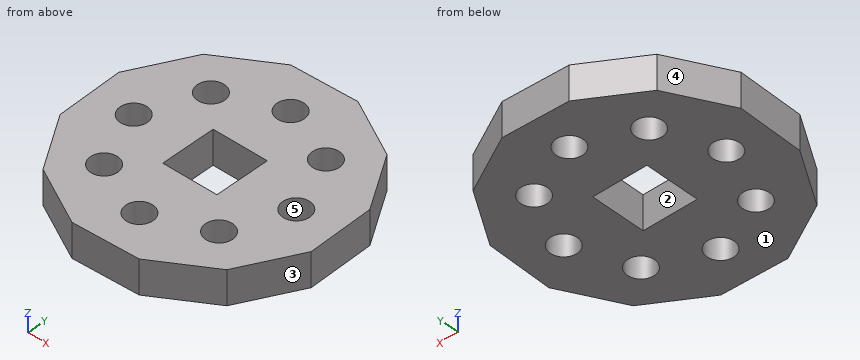
from build123d import *

# Parameters (mm, degrees)
SKETCH3_R           = 10
SKETCH3_W           = 40
SKETCH3_H           = 40
BOSS_EXTRUDE1_DEPTH = 25


with BuildPart() as part:
    # Sketch3 → Boss-Extrude1 (new body)
    with BuildSketch(Plane.XY):
        Polygon((21.199617339, 90.731086511), (-27.006136089, 89.175234501), (-67.975617162, 63.724950422), (-90.731086511, 21.199617339), (-89.175234501, -27.006136089), (-63.724950422, -67.975617162), (-21.199617339, -90.731086511), (27.006136089, -89.175234501), (67.975617162, -63.724950422), (90.731086511, -21.199617339), (89.175234501, 27.006136089), (63.724950422, 67.975617162), align=None)
        with Locations((0, 60)):
            Circle(SKETCH3_R, mode=Mode.SUBTRACT)
        with Locations((42.426406871, 42.426406871)):
            Circle(SKETCH3_R, mode=Mode.SUBTRACT)
        with Locations((60, 0)):
            Circle(SKETCH3_R, mode=Mode.SUBTRACT)
        with Locations((42.426406871, -42.426406871)):
            Circle(SKETCH3_R, mode=Mode.SUBTRACT)
        with Locations((0, -60)):
            Circle(SKETCH3_R, mode=Mode.SUBTRACT)
        with Locations((-42.426406871, -42.426406871)):
            Circle(SKETCH3_R, mode=Mode.SUBTRACT)
        with Locations((-60, 0)):
            Circle(SKETCH3_R, mode=Mode.SUBTRACT)
        with Locations((-42.426406871, 42.426406871)):
            Circle(SKETCH3_R, mode=Mode.SUBTRACT)
        Rectangle(SKETCH3_W, SKETCH3_H, mode=Mode.SUBTRACT)
    extrude(amount=BOSS_EXTRUDE1_DEPTH)


solid = part.part
Work out the finished part from the listing and answer in its coordinate system (mm). Face numbers are marked on the shaded views. A direction names the side the tool comes from. Round coordinates to 2 decimals unless told otherwise and drop trailing zeros. Write each loop counter-clockwise with the first axis right and the second up, starting at its lowest first coordinate (ties: lowest second). Pieces come first, ordered by that corner, then holes.
1) A cutting plane is placed at C-C (z = 3.75). Give the number of separate pieces and of enclosed holes in the cut face, plus the area to 3 significant figures.
2) Straight lines are drawn through the part: line 1 (Y direction, x = 44.5, z = 13.5); line 2 (X direction, y = 44, z = 23.75); line 3 (Y direction, x = 0, z = 9.25). For each, find the intervals that lie inside material, in ascending order.
3) A cutting plane is placed at D-D (y = -60). Give the vertices of the cut face in (x, z).
4) A cutting plane is placed at B-B (x = 2.5). Give the vertices of the cut face in (y, z).
5) Given pin 1 Ø18 at (x, y) = (-60, 0) entering from -Z; pin 2 Ø8 at (x, z) = (30.5, 21) entering from +Y; pin 3 Ø1 at (y, z) = (-57.5, 11) entering from -X; pin 4 Ø12 at (y, z) = (38, 5.5) entering from +X, each flat-ended and moving along its own axis, determine where each tip first touches the part or whether it passes through.
6) The mould has two halves that part along X. Classify the marked faces 3, 4 and 5: pulls with the +X half, pulls with the -X half, needs draft (parallel to the pull), parting line crosses it, or undercut.
7) A cutting plane is placed at A-A (x = -36.5). Give the vertices of the cut face in (y, z), plus the area to 3 significant figures.
8) A tool of negligible diameter and unlimited length cuts with its end or side. For the marked faces 1 and 2, from which of +Z, -Z, +X, -X, +Y, -Y can it reach the whole face along a straight path? Write none if from no direction.
Completed:
1. separate pieces: 1
1. enclosed holes: 9
1. area: 21,900 mm2
2. line 1: y = -78.31 to -52.21, -32.64 to 32.64, 52.21 to 78.26
2. line 2: x = -78.53 to -52.3, -32.55 to 32.55, 52.3 to 78.62
2. line 3: y = -90.05 to -70, -50 to -20, 20 to 50, 70 to 90.05
3. outline: (-68.68, 0) - (-10, 0) - (-10, 25) - (-68.68, 25) - close; (10, 0) - (69.97, 0) - (69.97, 25) - (10, 25) - close
4. outline: (-89.97, 0) - (-69.68, 0) - (-69.68, 25) - (-89.97, 25) - close; (-50.32, 0) - (-20, 0) - (-20, 25) - (-50.32, 25) - close; (20, 0) - (50.32, 0) - (50.32, 25) - (20, 25) - close; (69.68, 0) - (90.13, 0) - (90.13, 25) - (69.68, 25) - close
5. pin 1: passes through
5. pin 2: stops at y = 87.89
5. pin 3: stops at x = -70.54
5. pin 4: stops at x = 86.07
6. face 3: pulls with the +X half
6. face 4: pulls with the -X half
6. face 5: undercut
7. outline: (-82.54, 0) - (-50.48, 0) - (-50.48, 25) - (-82.54, 25) - close; (-34.37, 0) - (34.37, 0) - (34.37, 25) - (-34.37, 25) - close; (50.48, 0) - (83.28, 0) - (83.28, 25) - (50.48, 25) - close
7. area: 3,340 mm2
8. face 1: -Z, +X, -X, +Y, -Y
8. face 2: +Z, -Z
